Model file for the job. Use its own axes, mm. Face numbers are marked on the shaded views. Give positions to 0.01 mm unless a question says otherwise; leave off trailing zeros. Write each loop counter-clockwise with the first axis right and the second up, starting at its lowest first coordinate (ties: lowest second). Pieces come first, ordered by that corner, then holes. Notation, with made-up numbers: (-31.5, 46) - (8.5, 46) arc R12 ccw to (8.5, 68) - close; hole circle Ø1 at (2.5, 24.25). An arc over 180 degrees is marked (long way). One line per item, written item: value. Start each with the question number.
(1) Cut at C-C, the plane z = 11.5. List the corners of the cut face in (x, y), and give its area (3 significant figures).
(2) Cut at A-A, the plane y = -10.6. List the corners of the cut face in (x, z), and give its area (3 significant figures).
(3) Cut at B-B, the plane x = 89. List the corners of the cut face in (y, z), and give its area (3 significant figures).
(4) Drop flat-ended pins along their axis: P1, Ø0.6, axis at x = 92.5, z = 0, coming from the -Y side; P2, Ø4, axis at x = 87, y = -11, coming from the +Z side; P3, Ø3, axis at y = -1, z = 7.5, coming from the +X side (3 decimals). Give the stop position or say it passes through.
(5) Mould opens along Y. For the marked faces 1, 2, 3 and 4 say: pulls with the +Y half, pulls with the -Y half, needs draft (parallel to the pull), parting line crosses it, or undercut.
(6) Cut at D-D, the plane x = 84. List the corners of the cut face in (y, z), and give its area (3 significant figures).
(7) Probe L1, parallel to Y at x = 89, z = 15.7; L2, parallel to X at y = -10.6, z = 15.1; L3, parallel to Z at x = 78.5, y = -0.75. List the from-to ranges inside material, lowest first.
from build123d import *

# Parameters (mm, degrees)
BOX007_W                  = 50
BOX007_H                  = 25
BOX007_DEPTH              = 0.5
CYLINDER007_R             = 4.15
CYLINDER007_DEPTH         = 10
SKETCH006_R               = 15
EXTRUDE003003_DEPTH       = 17.25
CUT005013_PLACEMENT_ANGLE = 90


with BuildPart() as cube007:
    # Box007 → Box007 (new body)
    with BuildSketch(Plane(origin=(66, -23, 0), x_dir=(1, 0, 0), z_dir=(0, 0, 1))):
        with Locations((25, 12.5)):
            Rectangle(BOX007_W, BOX007_H)
    extrude(amount=BOX007_DEPTH)


with BuildPart() as obj1:
    # Cylinder007 → Cylinder007 (new body)
    with BuildSketch(Plane(origin=(89, -14.3, 10.4), x_dir=(1, 0, 0), z_dir=(0, -1, 0))):
        Circle(CYLINDER007_R)
    extrude(amount=CYLINDER007_DEPTH)


with BuildPart() as obj2:
    # Sketch006 → Extrude003003 (new body)
    with BuildSketch(Plane.XZ):
        with Locations((89, 10.4)):
            Circle(SKETCH006_R)
    extrude(amount=EXTRUDE003003_DEPTH)

    # Cut005013: cut obj1
    add(obj1.part, mode=Mode.SUBTRACT)


with BuildPart() as obj2_1:
    # Cut005013 placement: moved
    add(obj2.part.moved(Location((0, -21, 0))).rotate(Axis((0, -21, 0), (-1, 0, 0)), CUT005013_PLACEMENT_ANGLE))

    # Cut005014: cut Cube007
    add(cube007.part, mode=Mode.SUBTRACT)


solid = obj2_1.part
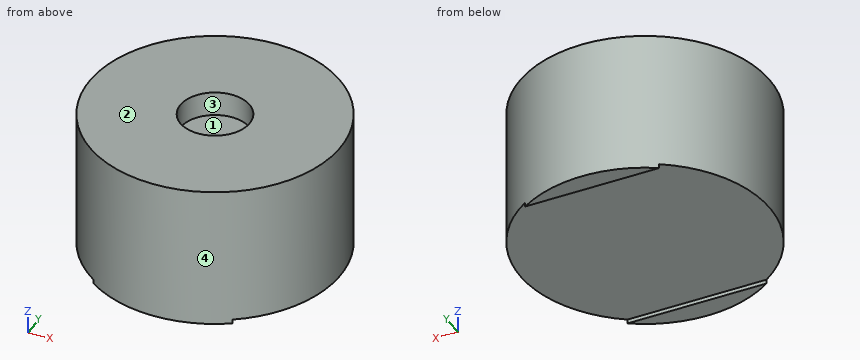
Answers follow:
1. outline: circle Ø30 at (89, -10.6)
1. area: 707 mm²
2. outline: (74, 0.5) - (104, 0.5) - (104, 17.25) - (93.15, 17.25) - (93.15, 14.3) - (84.85, 14.3) - (84.85, 17.25) - (74, 17.25) - close
2. area: 478 mm²
3. outline: (-25.6, 0) - (-23, 0) - (-23, 0.5) - (2, 0.5) - (2, 0) - (4.4, 0) - (4.4, 17.25) - (-6.45, 17.25) - (-6.45, 14.3) - (-14.75, 14.3) - (-14.75, 17.25) - (-25.6, 17.25) - close
3. area: 481 mm²
4. P1: stops at y = -25.25
4. P2: stops at z = 14.3
4. P3: stops at x = 101.625
5. face 1: undercut
5. face 2: needs draft
5. face 3: undercut
5. face 4: parting line crosses it
6. outline: (-24.74, 0) - (-23, 0) - (-23, 0.5) - (2, 0.5) - (2, 0) - (3.54, 0) - (3.54, 17.25) - (-24.74, 17.25) - close
6. area: 475 mm²
7. L1: y = -25.6 to -14.75, -6.45 to 4.4
7. L2: x = 74 to 84.85, 93.15 to 104
7. L3: z = 0.5 to 17.25
